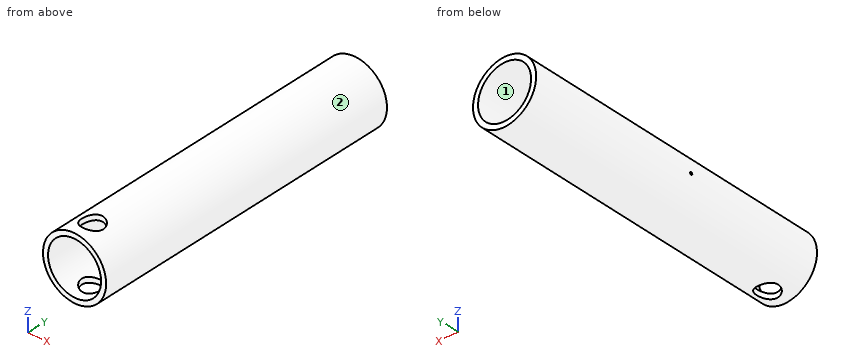
```python
from build123d import *

# Parameters (mm, degrees)
SKETCH_1_R               = 12.5
SKETCH_1_R_2             = 10.5
EXTRUDE_1_DEPTH          = 125
CUT_EXTRUDE_1_DEPTH      = 127.24381173
CUT_EXTRUDE_1_DEPTH_BACK = 127.24381173
SKETCH_2_R               = 4.25
SKETCH_4_R               = 0.5
CUT_EXTRUDE_3_DEPTH      = 25


with BuildPart() as part:
    # Эскиз1 → Бобышка-Вытянуть1 (new body)
    with BuildSketch(Plane(origin=(0, 0, 0), x_dir=(1, 0, 0), z_dir=(0, 1, 0))):
        with Locations(Location((0, 0, 0), (0, 0, 270))):
            Circle(SKETCH_1_R)
        with Locations(Location((0, 0, 0), (0, 0, 270))):
            Circle(SKETCH_1_R_2, mode=Mode.SUBTRACT)
    extrude(amount=EXTRUDE_1_DEPTH)

    # Эскиз2 → Вырез-Вытянуть1 (cut, two sides: drawn at the far end of the back side and taken through both)
    with BuildSketch(Plane.XY.offset(-CUT_EXTRUDE_1_DEPTH_BACK)):
        with Locations((0, 8)):
            Circle(SKETCH_2_R)
    extrude(amount=CUT_EXTRUDE_1_DEPTH + CUT_EXTRUDE_1_DEPTH_BACK, mode=Mode.SUBTRACT)

    # Эскиз4 → Вырез-Вытянуть3 (cut)
    with BuildSketch(Plane(origin=(0, 0, 0), x_dir=(0, 0, -1), z_dir=(1, 0, 0))):
        with Locations((0, 56)):
            Circle(SKETCH_4_R)
    extrude(amount=-CUT_EXTRUDE_3_DEPTH, mode=Mode.SUBTRACT)


solid = part.part
```
Geometry check sheet. Reference: the model listing, model coordinates, mm. Face numbers are marked on the shaded views. Round coordinates to 2 decimals unless told otherwise and drop trailing zeros. Loops run counter-clockwise (first coordinate to the right, second up) from the corner with the lowest first, then second, coordinate; pieces in that order, holes last. Notation, with made-up numbers: (-31.5, 49) - (6.5, 49) arc R20 cw to (6.5, 69) - close; hole circle Ø1 at (-31, 34.5). An arc over 180 degrees is marked (long way). Write each question's results on one line, items separated by ' | '. Start each with the question number.
Q1. Release check for a two-part mould opening along Z. For the marked faces 1 and 2 record: +Z half, -Z half, draft (parallel to the pull), parting line (faces both ways), or undercut.
Q2. Thickness scan on line 1 (Y direction, x = 0, z = 11.95); line 2 (Z direction, x = 0, y = 22.5); line 3 (X direction, y = 50, z = -4). Record the ranges inside material, lowest first. Write a range as [from, to].
Q3. Cross-section at A-A on x = 0. Enter the section's corners in (y, z), and give its area (3 significant figures).
Q4. Gauge pin test, flat ends, axial feed: P1, Ø10, axis at y = 101, z = 6.5, coming from the +X side; P2, Ø1, axis at y = 112.5, z = -6.5, coming from the +X side; P3, Ø2, axis at y = 40, z = -9, coming from the +X side. Record the tip position at first contact, or that the pin passes through.
Q5. Cross-section at B-B on y = 11. Enter the section's corners in (x, z), and give its area (3 significant figures).
Q6. Cross-section at C-C on z = 7.25. Enter the section's corners in (x, y).
Q7. Cross-section at D-D on y = 58.5. Enter the section's corners in (x, z).
Answers below:
1) face 1: undercut | face 2: parting line
2) line 1: y = [0, 3.75], [12.25, 125] | line 2: z = [-12.5, -10.5], [10.5, 12.5] | line 3: x = [-11.84, -9.71], [9.71, 11.84]
3) outline: (0, -12.5) - (3.75, -12.5) - (3.75, -10.5) - (0, -10.5) - close; (0, 10.5) - (3.75, 10.5) - (3.75, 12.5) - (0, 12.5) - close; (12.25, -12.5) - (125, -12.5) - (125, -10.5) - (12.25, -10.5) - close; (12.25, 10.5) - (125, 10.5) - (125, 12.5) - (12.25, 12.5) - close | area: 466 mm²
4) P1: stops at x = 12.41 | P2: stops at x = 10.97 | P3: stops at x = 9.6
5) outline: (-3.01, -12.13) - (-3.01, -10.06) arc R10.5 cw to (-3.01, 10.06) - (-3.01, 12.13) arc R12.5 ccw to start; (3.01, -12.13) arc R12.5 ccw to (3.01, 12.13) - (3.01, 10.06) arc R10.5 cw to (3.01, -10.06) - close | area: 120 mm²
6) outline: (-10.18, 0) - (-7.6, 0) - (-7.6, 125) - (-10.18, 125) - close; (7.6, 0) - (10.18, 0) - (10.18, 125) - (7.6, 125) - close
7) outline: circle Ø25 at (0, 0); hole circle Ø21 at (0, 0)
